```python
from build123d import *

# Parameters (mm, degrees)
SKETCH1_W           = 9.4
SKETCH1_H           = 16.5
BOSS_EXTRUDE1_DEPTH = 0.3
SKETCH2_W           = 5
SKETCH2_H           = 5
BOSS_EXTRUDE2_DEPTH = 1.5
CUT_EXTRUDE1_DEPTH  = 0.01
LPATTERN1_COUNT     = 4
LPATTERN1_PITCH     = 16.5


with BuildPart() as part:
    # Sketch1 → Boss-Extrude1 (new body)
    with BuildSketch(Plane(origin=(0, 0, 0), x_dir=(1, 0, 0), z_dir=(0, 1, 0))):
        Rectangle(SKETCH1_W, SKETCH1_H)
    boss_extrude1 = extrude(amount=BOSS_EXTRUDE1_DEPTH)

    # Sketch2 → Boss-Extrude2 (add)
    with BuildSketch(Plane(origin=(0, 0.3, 0), x_dir=(1, 0, 0), z_dir=(0, 1, 0))):
        with Locations((0, -0.3)):
            Rectangle(SKETCH2_W, SKETCH2_H)
    boss_extrude2 = extrude(amount=BOSS_EXTRUDE2_DEPTH)

    # Sketch3 → Cut-Extrude1 (cut)
    with BuildSketch(Plane(origin=(0, 0.3, 0), x_dir=(1, 0, 0), z_dir=(0, 1, 0))):
        Polygon((-0.34778048, 5.281417879), (-0.79778048, 5.281417879), (0, 4.281417879), (0.80221952, 5.251170562), (0.35221952, 5.251170562), (0.35221952, 7.651170562), (-0.34778048, 7.651170562), align=None)
    cut_extrude1 = extrude(amount=-CUT_EXTRUDE1_DEPTH, mode=Mode.SUBTRACT)

    # LPattern1: Boss-Extrude1, Boss-Extrude2, Cut-Extrude1 ×4
    with Locations(*[(0, 0, i * LPATTERN1_PITCH) for i in range(1, LPATTERN1_COUNT)]):
        add(boss_extrude1)
        add(boss_extrude2)
        add(cut_extrude1, mode=Mode.SUBTRACT)


solid = part.part
```
Could you check a few things on this model? Use its own coordinates, in mm. A direction names the side the tool comes from. Give positions to 0.01 mm unless a question says otherwise; leave off trailing zeros. Write each loop counter-clockwise with the first axis right and the second up, starting at its lowest first coordinate (ties: lowest second). Pieces come first, ordered by that corner, then holes. Notation, with made-up numbers: (-30, 5) -> (-6, 5) arc R8 cw to (-6, 12) -> close; hole circle Ø9 at (58, -1.75). An arc over 180 degrees is marked (long way). Write each question's results on one line, items separated by ' | '.
1. I want a section at D-D, the plane z = 8. Write out the boundary of the cut face in (x, y).
Check sheet entries:
outline: (-4.7, 0) -> (4.7, 0) -> (4.7, 0.3) -> (-4.7, 0.3) -> close
2. If we mould it in two halves opening along Z, with no side actions, what happens to faces 4 (the flat face through (0, 1, 19.3)), 5 (the flat face through (0, 1, 52.3)), 6 (the flat face through (2.5, 1, 17)), 7 (the flat face through (0, 1, -2.2))? For each: released by +Z, released by -Z, zero draft, split by the parting line, or undercut.
Check sheet entries:
face 4: undercut | face 5: released by +Z | face 6: zero draft | face 7: released by -Z
3. I want a section at B-B, the plane z = 17. Write out the boundary of the cut face in (x, y), then the cut area to 3 significant figures.
Check sheet entries:
outline: (-4.7, 0) -> (4.7, 0) -> (4.7, 0.3) -> (2.5, 0.3) -> (2.5, 1.8) -> (-2.5, 1.8) -> (-2.5, 0.3) -> (-4.7, 0.3) -> close | area: 10.3 mm²
4. I want a section at A-A, the plane y = 0.6. Write out the boundary of the cut face in (x, z).
Check sheet entries:
outline: (-2.5, -2.2) -> (2.5, -2.2) -> (2.5, 2.8) -> (-2.5, 2.8) -> close; (-2.5, 14.3) -> (2.5, 14.3) -> (2.5, 19.3) -> (-2.5, 19.3) -> close; (-2.5, 30.8) -> (2.5, 30.8) -> (2.5, 35.8) -> (-2.5, 35.8) -> close; (-2.5, 47.3) -> (2.5, 47.3) -> (2.5, 52.3) -> (-2.5, 52.3) -> close
5. Will these pins go through, and if not, where does the flat tip stop? pin 1 Ø0.5 at (x, z) = (-0.5, 44) entering from +Y; pin 2 Ø0.8 at (x, y) = (1, 1) entering from +Z.
Check sheet entries:
pin 1: stops at y = 0.3 | pin 2: stops at z = 52.3
6. On a 3-axis mill with a long thin cutter (end or side, diameter ignored), from which of +Z, -Z, +X, -X, +Y, -Y can I reach the whole of each face in a straight line? I mean faces 1 (the flat face through (2.5, 1, 50)), 2 (the flat face through (0, 1, 30.8)), 3 (the flat face through (-2.5, 1, 0)). Say none if no direction works.
Check sheet entries:
face 1: +Z, -Z, +X, +Y | face 2: +X, -X, +Y | face 3: +Z, -Z, -X, +Y
7. I want a section at C-C, the plane x = 4. Write out the boundary of the cut face in (y, z).
Check sheet entries:
outline: (0, -8.25) -> (0.3, -8.25) -> (0.3, 57.75) -> (0, 57.75) -> close
8. I need wall thicknesses on L1, parallel to Z at x = -0.5, y = 1.45; L2, parallel to Y at x = -3.75, z = 23; L3, parallel to X at y = 0.4, z = 2. Which ranges of each line are inside material? Lowest first, please.
Check sheet entries:
L1: z = -2.2 to 2.8, 14.3 to 19.3, 30.8 to 35.8, 47.3 to 52.3 | L2: y = 0 to 0.3 | L3: x = -2.5 to 2.5
